Could you check a few things on this model? Use its own coordinates, in mm. Round coordinates to 2 decimals unless told otherwise and drop trailing zeros. Loops run counter-clockwise (first coordinate to the right, second up) from the corner with the lowest first, then second, coordinate; pieces in that order, holes last. Notation, with made-up numbers: (10.5, 67.25) -> (40.5, 67.25) arc R11 cw to (40.5, 71.25) -> close; hole circle Ø8 at (-18.75, 13). An arc over 180 degrees is marked (long way). Put each result on its own line as item: value. Start each with the question number.
1. Imagine slicing it at D-D, the plane x = 230. Please give me the cut outline in (y, z), and give its area (3 significant figures).
2. I'm going to push flat-ended pins straight in: P1, Ø13, axis at x = 69, y = 20, coming from the +Z side; P2, Ø8, axis at x = 115.5, y = 8, coming from the +Z side; P3, Ø3.5, axis at x = 184, z = -2, coming from the +Y side. Where does each tip first touch, or does it pass through?
3. I need wall thicknesses on line 1 (Y direction, x = 152.4, z = 1.6); line 2 (Y direction, x = 139.7, z = 1.05); line 3 (Z direction, x = 268.5, y = 42). Which ranges of each line are inside material? Lowest first, please. Write a range as [from, to].
4. Imagine slicing it at C-C, the plane y = 40. Please give me the cut outline in (x, z), and give its area (3 significant figures).
5. Imagine slicing it at B-B, the plane x = 42.5. Please give me the cut outline in (y, z), and give its area (3 significant figures).
6. Imagine slicing it at A-A, the plane z = 9.5. Please give me the cut outline in (x, y) (1 decimal), and give its area (3 significant figures).
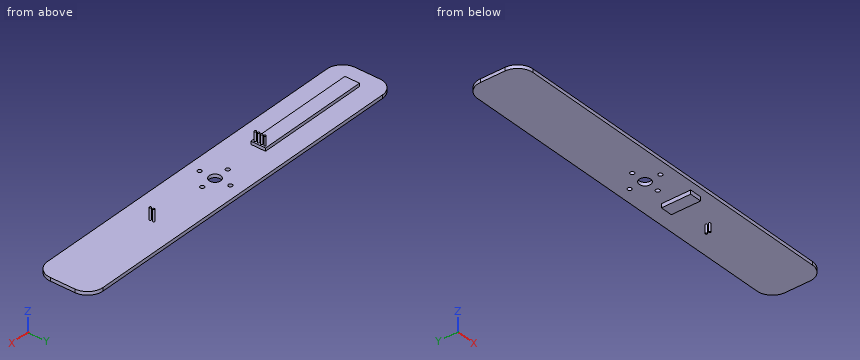
Autodesk Inventor part; units mm, degrees
ref_plane "YZ Plane" through (0, 0, 0) normal (1, 0, 0) x (0, 1, 0)
ref_plane "XZ Plane" through (0, 0, 0) normal (0, 1, 0) x (-1, 0, 0)
ref_plane "XY Plane" through (0, 0, 0) normal (0, 0, 1) x (1, 0, 0)
sketch "Sketch1" plane through (0, 0, 0) normal (0, 0, 1) x (1, 0, 0)
  line L0 (0, 0) -> (304.8, 0)
  line L1 (304.8, 0) -> (304.8, 45.72)
  line L2 (304.8, 45.72) -> (0, 45.72)
  line L3 (0, 45.72) -> (0, 0)
  dimension "d0" = 304.8
  dimension "d1" = 45.72
extrude "Extrusion1" add sketch "Sketch1" along normal blind 2.794
sketch "Sketch2" plane through (0, 0, 2.794) normal (0, 0, 1) x (1, 0, 0)
  line L0 (114.3, 0) -> (190.5, 0)
  line L1 (190.5, 0) -> (190.5, 35.56)
  line L2 (190.5, 35.56) -> (114.3, 35.56)
  line L3 (114.3, 35.56) -> (114.3, 0)
  line L4 (114.3, 0) -> (190.5, 35.56) construction
  line L5 (190.5, 0) -> (114.3, 35.56) construction
  line L6 (108.6972, 16.51) -> (14.7172, 16.51)
  line L7 (14.7172, 16.51) -> (14.7172, 28.5496)
  line L8 (14.7172, 28.5496) -> (108.6972, 28.5496)
  line L9 (108.6972, 28.5496) -> (108.6972, 16.51)
  line L10 (108.6972, 16.51) -> (14.7172, 28.5496) construction
  line L11 (14.7172, 16.51) -> (108.6972, 28.5496) construction
  circle A0 centre (106.812, 26.4905) radius 0.7825
  line L12 (14.7172, 13.843) -> (108.6972, 25.8826) construction
  circle A1 centre (106.812, 23.8235) radius 0.7825
  line L13 (14.7172, 11.176) -> (108.6972, 23.2156) construction
  circle A2 centre (106.812, 21.1565) radius 0.7825
  line L14 (14.7172, 8.509) -> (108.6972, 20.5486) construction
  circle A3 centre (106.812, 18.4895) radius 0.7825
  line L15 (0, 0) -> (304.8, 0)
  line L16 (0, 45.72) -> (0, 0)
  point P0 (152.4, 17.78)
  point P1 (61.7072, 22.5298)
  dimension "d4" = 76.2
  dimension "d5" = 35.56
  dimension "d6" = 93.98
  dimension "d7" = 12.0396
  dimension "d10" = 2.667
  dimension "d56" = 16.51
  dimension "d57" = 14.7172
  dimension "d58" = 2.0591
  dimension "d59" = 1.8853
  dimension "d60" = 1.102
extrude "Extrusion2" add sketch "Sketch2" along normal blind 10.16 contours A0 | A1 | A2 | A3
sketch "Sketch3" plane through (0, 0, 2.794) normal (0, 0, 1) x (1, 0, 0)
  line L0 (114.3, 0) -> (190.5, 0)
  line L1 (190.5, 0) -> (190.5, 35.56)
  line L2 (190.5, 35.56) -> (114.3, 35.56)
  line L3 (114.3, 35.56) -> (114.3, 0)
  line L4 (114.3, 0) -> (190.5, 35.56) construction
  line L5 (190.5, 0) -> (114.3, 35.56) construction
  line L6 (108.6972, 16.4402) -> (14.7172, 16.4401)
  line L7 (14.7172, 16.4401) -> (14.7172, 28.4797)
  line L8 (14.7172, 28.4797) -> (108.6972, 28.4798)
  line L9 (108.6972, 28.4798) -> (108.6972, 16.4402)
  line L10 (108.6972, 16.4402) -> (14.7172, 28.4797) construction
  line L11 (14.7172, 16.4401) -> (108.6972, 28.4798) construction
  circle A0 centre (106.812, 26.4207) radius 0.7825
  line L12 (14.7172, 13.7731) -> (108.6972, 25.8128) construction
  circle A1 centre (106.812, 23.7537) radius 0.7825
  line L13 (14.7172, 11.1061) -> (108.6972, 23.1458) construction
  circle A2 centre (106.812, 21.0867) radius 0.7825
  line L14 (14.7172, 8.4391) -> (108.6972, 20.4788) construction
  circle A3 centre (106.812, 18.4197) radius 0.7825
  line L15 (304.8, 45.72) -> (0, 45.72)
  line L16 (0, 45.72) -> (0, 0)
  line L17 (0, 0) -> (304.8, 0)
  point P0 (152.4, 17.78)
  dimension "d17" = 76.2
  dimension "d18" = 35.56
  dimension "d19" = 93.98
  dimension "d20" = 12.0396
  dimension "d21" = 2.667
  dimension "d63" = 2.0591
  dimension "d64" = 1.8853
  dimension "d68" = 16.4401
extrude "Extrusion3" add sketch "Sketch3" along normal blind 2.54 contours L6 L7 L8 L9
sketch "Sketch5" plane through (0, 0, 2.794) normal (0, 0, 1) x (1, 0, 0)
  circle A0 centre (106.812, 23.8235) radius 0.7825
  circle A1 centre (106.812, 21.1565) radius 0.7825
  circle A2 centre (214.4081, 23.402) radius 0.7825
  circle A3 centre (214.4081, 20.735) radius 0.7825
  line L0 (108.6972, 16.4402) -> (108.6972, 28.4798)
  point P0 (0, 0)
  dimension "d65" = 107.5969
  dimension "d66" = 105.7108
  dimension "d67" = 107.5961
extrude "Extrusion4" add sketch "Sketch5" along normal mid plane 19.05 contours A2 | A3
sketch "Sketch6" plane through (0, 0, 2.794) normal (0, 0, 1) x (1, 0, 0)
  circle A0 centre (152.4, 35.56) radius 1.6891
  circle A1 centre (152.4, 10.16) radius 1.6891
  circle A2 centre (165.1, 22.86) radius 1.6891
  circle A3 centre (139.7, 22.86) radius 1.6891
  circle A4 centre (152.4, 22.86) radius 4.699
  line L0 (304.8, 45.72) -> (0, 45.72)
  line L1 (0, 45.72) -> (0, 0)
  dimension "d37" = 3.3782
  dimension "d38" = 3.3782
  dimension "d39" = 3.3782
  dimension "d40" = 3.3782
  dimension "d47" = 9.398
  dimension "d78" = 12.7
  dimension "d79" = 12.7
  dimension "d81" = 12.7
  dimension "d82" = 12.7
  dimension "d83" = 0
extrude "Extrusion5" cut sketch "Sketch6" against normal blind 8.89
fillet "Fillet1" radius 12.7 4 edges at (304.8, 0, 1.397) (304.8, 45.72, 1.397) (0, 0, 1.397) (0, 45.72, 1.397)
sketch "Sketch8" plane through (0, 0, 0) normal (0, 0, -1) x (-1, 0, 0)
  line L0 (-177.9476, 6.2522) -> (-187.8536, 6.2522)
  line L1 (-187.8536, 6.2522) -> (-187.8536, 30.3822)
  line L2 (-187.8536, 30.3822) -> (-177.9476, 30.3822)
  line L3 (-177.9476, 30.3822) -> (-177.9476, 6.2522)
  point P0 (0, 0)
  dimension "d48" = 9.906
  dimension "d49" = 24.13
extrude "Extrusion6" add sketch "Sketch8" along normal blind 3.2258
sketch "Sketch9" plane through (0, 0, 2.794) normal (0, 0, 1) x (1, 0, 0)
  line L0 (102.87, 1.27) -> (217.17, 1.27)
  line L1 (217.17, 1.27) -> (217.17, 44.45)
  line L2 (217.17, 44.45) -> (102.87, 44.45)
  line L3 (102.87, 44.45) -> (102.87, 1.27)
  line L4 (102.87, 1.27) -> (217.17, 44.45) construction
  line L5 (217.17, 1.27) -> (102.87, 44.45) construction
  line L6 (12.7, 0) -> (292.1, 0)
  line L7 (304.8, 12.7) -> (304.8, 33.02)
  point P0 (160.02, 22.86)
  dimension "d69" = 114.3
  dimension "d70" = 43.18
  dimension "d76" = 44.45
  dimension "d77" = 87.63
properties part number "Base"
Entries:
1. outline: (0, 0) -> (45.72, 0) -> (45.72, 2.79) -> (0, 2.79) -> close
1. area: 128 mm^2
2. P1: z = 5.33
2. P2: z = 2.79
2. P3: y = 30.38
3. line 1: [0, 8.47], [11.85, 18.16], [27.56, 33.87], [37.25, 45.72]
3. line 2: [0, 21.17], [24.55, 45.72]
3. line 3: [0, 2.79]
4. outline: (2.09, 0) -> (302.71, 0) -> (302.71, 2.79) -> (2.09, 2.79) -> close
4. area: 840 mm^2
5. outline: (0, 0) -> (45.72, 0) -> (45.72, 2.79) -> (28.48, 2.79) -> (28.48, 5.33) -> (16.44, 5.33) -> (16.44, 2.79) -> (0, 2.79) -> close
5. area: 158 mm^2
6. outline: circle Ø1.6 at (106.8, 18.5); circle Ø1.6 at (106.8, 21.2); circle Ø1.6 at (106.8, 23.8); circle Ø1.6 at (106.8, 26.5); circle Ø1.6 at (214.4, 20.7); circle Ø1.6 at (214.4, 23.4)
6. area: 11.5 mm^2
